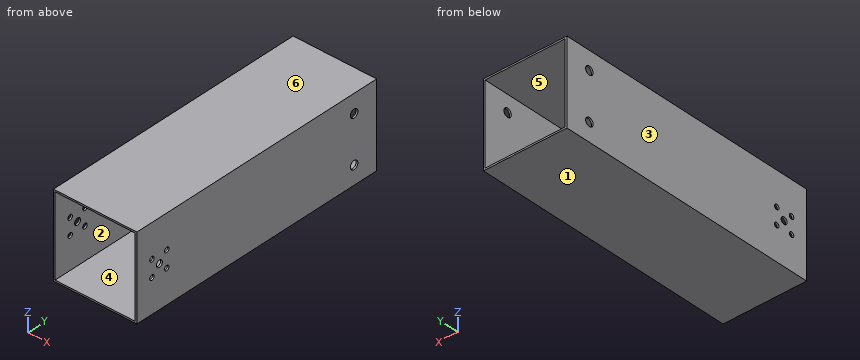
Autodesk Inventor part; units mm, degrees
ref_plane "YZ Plane" through (0, 0, 0) normal (1, 0, 0) x (0, 1, 0)
ref_plane "XZ Plane" through (0, 0, 0) normal (0, 1, 0) x (-1, 0, 0)
ref_plane "XY Plane" through (0, 0, 0) normal (0, 0, 1) x (1, 0, 0)
sketch "Sketch1" plane through (0, 0, 0) normal (0, 1, 0) x (-1, 0, 0)
  line L0 (25, 25) -> (-25, 25)
  line L1 (-25, 25) -> (-25, -25)
  line L2 (-25, -25) -> (25, -25)
  line L3 (25, -25) -> (25, 25)
  line L4 (25, 25) -> (-25, -25) construction
  line L5 (-25, 25) -> (25, -25) construction
  line L6 (24, 24) -> (-24, 24)
  line L7 (-24, 24) -> (-24, -24)
  line L8 (-24, -24) -> (24, -24)
  line L9 (24, -24) -> (24, 24)
  line L10 (24, 24) -> (-24, -24) construction
  line L11 (-24, 24) -> (24, -24) construction
  point P0 (0, 0)
  dimension "d0" = 50
  dimension "d2" = 48
extrude "Extrusion1" add sketch "Sketch1" along normal blind 160
sketch "Sketch2" plane through (25, 0, 25) normal (1, 0, 0) x (0, 0, -1)
  line L0 (0, 0) -> (48, 0) construction
  line L1 (0, 0) -> (0, 15) construction
  line L2 (0, 15) -> (11, 15) construction
  line L3 (11, 15) -> (39, 15) construction
  line L4 (25, 15) -> (20.0503, 19.9497) construction
  line L5 (25, 15) -> (32, 15) construction
  line L6 (20.0503, 19.9497) -> (20.0503, 22.4497) construction
  line L7 (21.4936, 22.4497) -> (22.937, 19.9497)
  line L8 (22.937, 19.9497) -> (21.4936, 17.4497)
  line L9 (21.4936, 17.4497) -> (18.6069, 17.4497)
  line L10 (18.6069, 17.4497) -> (17.1635, 19.9497)
  line L11 (17.1635, 19.9497) -> (18.6069, 22.4497)
  line L12 (18.6069, 22.4497) -> (21.4936, 22.4497)
  line L13 (25, 15) -> (25, 18.7194) construction
  circle A0 centre (20.0503, 19.9497) radius 1.5
  line L14 (29.9497, 19.9497) -> (29.9497, 22.4497) construction
  line L15 (28.5064, 22.4497) -> (27.063, 19.9497)
  line L16 (27.063, 19.9497) -> (28.5064, 17.4497)
  line L17 (28.5064, 17.4497) -> (31.3931, 17.4497)
  line L18 (31.3931, 22.4497) -> (28.5064, 22.4497)
  line L19 (32.8365, 19.9497) -> (31.3931, 22.4497)
  line L20 (31.3931, 17.4497) -> (32.8365, 19.9497)
  circle A1 centre (29.9497, 19.9497) radius 1.5
  line L21 (20.0503, 10.0503) -> (20.0503, 7.5503) construction
  line L22 (21.4936, 7.5503) -> (22.937, 10.0503)
  line L23 (22.937, 10.0503) -> (21.4936, 12.5503)
  line L24 (21.4936, 12.5503) -> (18.6069, 12.5503)
  line L25 (18.6069, 7.5503) -> (21.4936, 7.5503)
  line L26 (17.1635, 10.0503) -> (18.6069, 7.5503)
  line L27 (18.6069, 12.5503) -> (17.1635, 10.0503)
  circle A2 centre (20.0503, 10.0503) radius 1.5
  line L28 (27.063, 10.0503) -> (28.5064, 12.5503)
  line L29 (28.5064, 12.5503) -> (31.3931, 12.5503)
  line L30 (28.5064, 7.5503) -> (27.063, 10.0503)
  circle A3 centre (29.9497, 10.0503) radius 1.5
  line L31 (31.3931, 12.5503) -> (32.8365, 10.0503)
  line L32 (31.3931, 7.5503) -> (28.5064, 7.5503)
  line L33 (32.8365, 10.0503) -> (31.3931, 7.5503)
  line L34 (29.9497, 10.0503) -> (29.9497, 7.5503) construction
  line L35 (0, 15) -> (0, 30) construction
  line L36 (0, 0) -> (0, 160) construction
  line L37 (25, 145) -> (32, 145) construction
  circle A4 centre (39, 145) radius 2.5
  line L38 (11, 145) -> (39, 145) construction
  line L39 (0, 130) -> (48, 130) construction
  line L40 (25, 145) -> (20.0503, 149.9497) construction
  line L41 (25, 145) -> (25, 148.7194) construction
  line L42 (0, 130) -> (0, 145) construction
  line L43 (0, 145) -> (11, 145) construction
  circle A5 centre (11, 145) radius 2.5
  line L44 (0, 145) -> (0, 160) construction
  circle A6 centre (25, 15) radius 2
  point P0 (25, 0)
  point P1 (25, 11.2806)
  dimension "d6" = 15
  dimension "d7" = 11
  dimension "d8" = 28
  dimension "d11" = 7
  dimension "d12" = 135
  dimension "d13" = 2.5
  dimension "d18" = 3
  dimension "d19" = 15
  dimension "d20" = 15
  dimension "d21" = 11
  dimension "d22" = 28
  dimension "d23" = 5
  dimension "d24" = 5
  dimension "d25" = 7
  dimension "d26" = 135
  dimension "d29" = 15
  dimension "d30" = 4
extrude "Extrusion2" cut sketch "Sketch2" against normal blind 50 contours A0 | A1 | A2 | A3 | A4 | A5 | A6
properties part number "End-Link" material "Aluminum 6061"
Source: CAD feature listing. Evaluate the final solid. Frame: model axes, mm. Face numbers are marked on the shaded views. A direction names the side the tool comes from. Coordinates: 2 decimals unless noted, no trailing zeros. Loops run counter-clockwise (first coordinate to the right, second up) from the corner with the lowest first, then second, coordinate; pieces in that order, holes last. Notation, with made-up numbers: M 21.25,-13.5 L 55.25,-13.5 A30 cw 55.25,15.5 Z; hole C 21,74.25 d4. An arc over 180 degrees is marked long. Put each result on its own line as item: value. Start each with the question number.
1) Cut plane B-B on z = -20.5. Return the cut outline in (x, y), then the cut area to 3 significant figures.
2) Reachability of the marked faces 1 and 2 from +Z, -Z, +X, -X, +Y, -Y: full face, straight path, thin tool, end or side. Return the list, or none.
3) Pull-direction query (Z, two-part tool) for the marked faces 3, 4, 5 and 6; classes: pulls with the +Z half, pulls with the -Z half, needs draft (parallel to the pull), parting line crosses it, or undercut.
4) Cut plane D-D on y = 37.5. Return the cut outline in (x, z), then the cut area to 3 significant figures.
5) Cut plane A-A on y = 145. Return the cut outline in (x, z).
6) Cut plane C-C on x = -6. Return the cut outline in (y, z).
7) Ray query, L1, parallel to X at y = 8.5, z = -14; L2, parallel to Z at x = 24.7, y = 145. Return the intervals inside material, ascending. Write a range as from..to.
The answers:
1. outline: M -25,0 L -24,0 L -24,160 L -25,160 Z; M 24,0 L 25,0 L 25,160 L 24,160 Z
1. area: 320 mm²
2. face 1: -Z, +X, -X, +Y, -Y
2. face 2: +Y, -Y
3. face 3: needs draft
3. face 4: undercut
3. face 5: undercut
3. face 6: pulls with the +Z half
4. outline: M -25,-25 L 25,-25 L 25,25 L -25,25 Z; hole M -24,-24 L 24,-24 L 24,24 L -24,24 Z
4. area: 196 mm²
5. outline: M -25,-25 L 25,-25 L 25,-16.5 L 24,-16.5 L 24,-24 L -24,-24 L -24,-16.5 L -25,-16.5 Z; M -25,-11.5 L -24,-11.5 L -24,11.5 L -25,11.5 Z; M -25,16.5 L -24,16.5 L -24,24 L 24,24 L 24,16.5 L 25,16.5 L 25,25 L -25,25 Z; M 24,-11.5 L 25,-11.5 L 25,11.5 L 24,11.5 Z
6. outline: M 0,-25 L 160,-25 L 160,-24 L 0,-24 Z; M 0,24 L 160,24 L 160,25 L 0,25 Z
7. L1: x = -25..-24, 24..25
7. L2: z = -25..-16.5, -11.5..11.5, 16.5..25
